Autodesk Inventor part; units mm, degrees
ref_plane "YZ Plane" through (0, 0, 0) normal (1, 0, 0) x (0, 1, 0)
ref_plane "XZ Plane" through (0, 0, 0) normal (0, 1, 0) x (-1, 0, 0)
ref_plane "XY Plane" through (0, 0, 0) normal (0, 0, 1) x (1, 0, 0)
sketch "Sketch1" plane through (0, 0, 0) normal (0, 0, 1) x (1, 0, 0)
  line L0 (-25, 25) -> (25, 25)
  line L1 (25, 25) -> (25, -25)
  line L2 (25, -25) -> (-25, -25)
  line L3 (-25, -25) -> (-25, 25)
  line L4 (-25, 25) -> (25, -25) construction
  line L5 (25, 25) -> (-25, -25) construction
  line L6 (0, 0) -> (-33.9411, 33.9411)
  circle A0 centre (-33.9411, 33.9411) radius 9
  line L7 (0, 0) -> (2.1213, 2.1213)
  line L8 (0, 0) -> (-2.1213, -2.1213)
  line L9 (2.1213, 2.1213) -> (-25.8198, 30.0624)
  line L10 (-2.1213, -2.1213) -> (-30.0624, 25.8198)
  line L11 (0, 0) -> (33.9411, -33.9411)
  circle A1 centre (33.9411, -33.9411) radius 9
  line L12 (2.1213, 2.1213) -> (30.0624, -25.8198)
  line L13 (-2.1213, -2.1213) -> (25.8198, -30.0624)
  line L14 (0, 25) -> (0, -25) construction
  line L15 (25, 25) -> (-25, 25)
  line L16 (-25, 25) -> (-25, -25)
  line L17 (-25, -25) -> (25, -25)
  line L18 (25, -25) -> (25, 25)
  line L19 (25, 25) -> (-25, -25) construction
  line L20 (-25, 25) -> (25, -25) construction
  line L21 (0, 0) -> (33.9411, 33.9411)
  circle A2 centre (33.9411, 33.9411) radius 9
  line L22 (0, 0) -> (-2.1213, 2.1213)
  line L23 (0, 0) -> (2.1213, -2.1213)
  line L24 (-2.1213, 2.1213) -> (25.8198, 30.0624)
  line L25 (2.1213, -2.1213) -> (30.0624, 25.8198)
  line L26 (0, 0) -> (-33.9411, -33.9411)
  circle A3 centre (-33.9411, -33.9411) radius 9
  line L27 (-2.1213, 2.1213) -> (-30.0624, -25.8198)
  line L28 (2.1213, -2.1213) -> (-25.8198, -30.0624)
  point P0 (-25, 20.7574)
  point P1 (-25, -20.7574)
  point P2 (-20.7574, -25)
  point P3 (20.7574, -25)
  point P4 (25, -20.7574)
  point P5 (25, 20.7574)
  point P6 (20.7574, 25)
  point P7 (-20.7574, 25)
  dimension "d0" = 50
  dimension "d1" = 50
  dimension "d5" = 48
  dimension "d6" = 18
  dimension "d7" = 3
  dimension "d8" = 3
extrude "Extrusion1" add sketch "Sketch1" along normal blind 5
sketch "Sketch2" plane through (0, 0, 5) normal (0, 0, 1) x (1, 0, 0)
  line L0 (-23, 23) -> (23, 23)
  line L1 (23, 23) -> (23, -23)
  line L2 (23, -23) -> (-23, -23)
  line L3 (-23, -23) -> (-23, 23)
  line L4 (-23, 23) -> (23, -23) construction
  line L5 (23, 23) -> (-23, -23) construction
  point P0 (0, 0)
  dimension "d11" = 46
  dimension "d12" = 46
extrude "Extrusion2" cut sketch "Sketch2" against normal blind 2
sketch "Sketch3" plane through (0, 0, 5) normal (0, 0, 1) x (1, 0, 0)
  arc A0 (-25.8198, 30.0624) -> (-30.0624, 25.8198) centre (-33.9411, 33.9411) ccw
  circle A1 centre (-33.9411, 33.9411) radius 8
  circle A2 centre (-33.9411, -33.9411) radius 8
  circle A3 centre (33.9411, -33.9411) radius 8
  circle A4 centre (33.9411, 33.9411) radius 8
  point P0 (0, 0)
  dimension "d15" = 16
  dimension "d18" = 360
extrude "Extrusion3" add sketch "Sketch3" along normal blind 1.5
properties part number "aruco_holder"
The listing builds one solid part. Answer for the finished solid, in the listing's coordinates (mm). A direction names the side the tool comes from. Round coordinates to 2 decimals unless told otherwise and drop trailing zeros. Order: outer loops, then holes, each group sorted by start corner. A loop starts at its lowest first (then second) coordinate and runs counter-clockwise, first axis right, second up. Notation, with made-up numbers: (38.5, -28.5) -> (93.5, -28.5) arc R24 cw to (93.5, 1.5) -> close; hole circle Ø8 at (86.5, 18.5). An arc over 180 degrees is marked (long way). One line per item, written item: value.
Item 1: Find section B-B, the plane z = 1.75. Give the vertices of the cut face in (x, y), then the cut area to 3 significant figures.
Taken from the geometry:
outline: (-30.06, -25.82) arc R9 ccw (long way) to (-25.82, -30.06) -> (-20.76, -25) -> (20.76, -25) -> (25.82, -30.06) arc R9 ccw (long way) to (30.06, -25.82) -> (25, -20.76) -> (25, 20.76) -> (30.06, 25.82) arc R9 ccw (long way) to (25.82, 30.06) -> (20.76, 25) -> (-20.76, 25) -> (-25.82, 30.06) arc R9 ccw (long way) to (-30.06, 25.82) -> (-25, 20.76) -> (-25, -20.76) -> close
area: 3,650 mm2
Item 2: Given P1, Ø1, axis at y = -1.5, z = 3, coming from the -X side; P2, Ø1, axis at x = 6.5, z = 4, coming from the -Y side; P3, Ø0.6, axis at y = 9, z = 4.5, coming from the +X side, each flat-ended and moving along its own axis, determine where each tip first touches the part or whether it passes through.
Taken from the geometry:
P1: stops at x = -25
P2: stops at y = -25
P3: stops at x = 25
Item 3: Straight lines are drawn through the part: L1, parallel to X at y = 2.5, z = 4.25; L2, parallel to X at y = -34.5, z = 2.5. For each, find the intervals that lie inside material, in ascending order.
Taken from the geometry:
L1: x = -25 to -23, 23 to 25
L2: x = -42.92 to -24.96, 24.96 to 42.92
Item 4: Find section C-C, the plane x = -36. Give the vertices of the cut face in (y, z), then the cut area to 3 significant figures.
Taken from the geometry:
outline: (-42.7, 0) -> (-25.18, 0) -> (-25.18, 5) -> (-26.21, 5) -> (-26.21, 6.5) -> (-41.67, 6.5) -> (-41.67, 5) -> (-42.7, 5) -> close; (25.18, 0) -> (42.7, 0) -> (42.7, 5) -> (41.67, 5) -> (41.67, 6.5) -> (26.21, 6.5) -> (26.21, 5) -> (25.18, 5) -> close
area: 222 mm2
Item 5: For faces 1 (the cylindrical face through (-41.933, 33.589, 5.74)), 2 (the flat face through (-34, 34, 6.5)), 3 (the cylindrical face through (40.05, 40.55, 2.46)), 4 (the flat face through (25, 0, 2)), 5 (the flat face through (0, 25, 2)), determine the directions among +Z, -Z, +X, -X, +Y, -Y from which every point of the face is accessible in a straight line to the end or side of a thin tool.
Taken from the geometry:
face 1: +Z
face 2: +Z, +X, -X, +Y, -Y
face 3: +Z, -Z
face 4: +Z, -Z, +X
face 5: +Z, -Z, +Y
Item 6: For a pull along X with two mould halves and no side action, classify faces 6 (the flat face through (-34, -34, 6.5)), 7 (the flat face through (23.253, 27.496, 2.465)), 8 (the flat face through (-25, 0, 2)) as released by +X, released by -X, zero draft, split by the parting line, or undercut.
Taken from the geometry:
face 6: zero draft
face 7: undercut
face 8: released by -X
Item 7: Find section A-A, the plane y = -1. Give the vertices of the cut face in (x, z), then the cut area to 3 significant figures.
Taken from the geometry:
outline: (-25, 0) -> (25, 0) -> (25, 5) -> (23, 5) -> (23, 3) -> (-23, 3) -> (-23, 5) -> (-25, 5) -> close
area: 158 mm2
